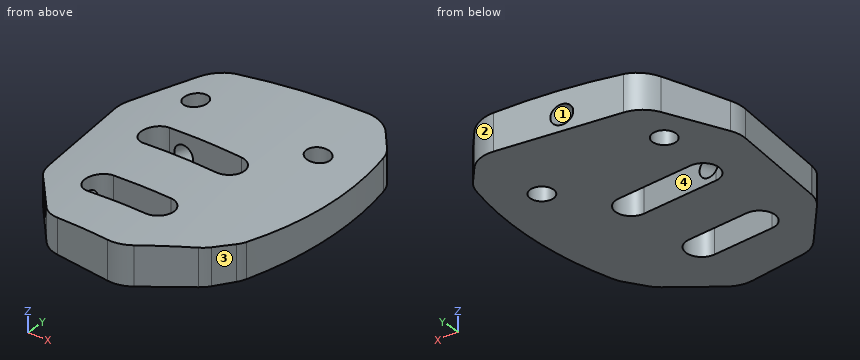
Autodesk Inventor part; units mm, degrees
ref_plane "ChannelAngleOrthoPlane" through (0.3382, 9.2918, 0) normal (-0.3338, -0.9426, 0) x (0, 0, 1)
ref_plane "YZ Plane" through (0, 0, 0) normal (1, 0, 0) x (0, 1, 0)
ref_plane "XZ Plane" through (0, 0, 0) normal (0, 1, 0) x (-1, 0, 0)
sketch "Base" plane through (0, 0, 0) normal (0, 0, 1) x (1, 0, 0)
  circle A0 centre (-15.6718, 1.2221) radius 1.5
  circle A1 centre (-13.9696, -18.0615) radius 2
  line L0 (-13.9696, -18.0615) -> (-6.0134, -18.8977) construction
  circle A2 centre (-6.0134, -18.8977) radius 2
  circle A3 centre (-14.8088, -6.9127) radius 2
  circle A4 centre (-4.8636, -7.958) radius 2
  line L1 (-14.8088, -6.9127) -> (-4.8636, -7.958) construction
  line L2 (-14.1786, -20.0505) -> (-6.2224, -20.8868)
  line L3 (-13.7605, -16.0724) -> (-5.8043, -16.9087)
  line L4 (-15.0178, -8.9017) -> (-5.0726, -9.947)
  line L5 (-14.5997, -4.9237) -> (-4.6545, -5.9689)
  line L6 (-6.0134, -18.8977) -> (-4.8636, -7.958) construction
  circle A5 centre (1.2351, -0.5549) radius 1.5
  line L7 (-15.6718, 1.2221) -> (1.2351, -0.5549) construction
  line L8 (-21.3231, -18.1609) -> (-22.5392, -2.7087)
  line L9 (-15.0979, -25.987) -> (-21.3231, -18.1609)
  line L10 (-22.5392, -2.7087) -> (-17.4079, 7.5831)
  line L11 (-17.4079, 7.5831) -> (2.5, 9.5)
  line L12 (-4.7419, -27.72) -> (2.6752, -22.6223)
  line L13 (-15.0979, -25.987) -> (-4.7419, -27.72)
  arc A6 (4.998, -19.3658) -> (6.2351, 4.8044) centre (-36.6314, -5.1184) ccw
  line L14 (2.6752, -22.6223) -> (4.998, -19.3658)
  line L15 (2.5, 9.5) -> (6.2351, 4.8044)
  line L16 (-45.5436, 0) -> (16.8418, 0) construction
  line L17 (0, -35.164) -> (0, 16.944) construction
  dimension "d119" = 8
  dimension "d129" = 10
  dimension "d290" = 11
  dimension "d293" = 3
  dimension "d294" = 122
  dimension "d295" = 123
  dimension "d296" = 149
  dimension "d297" = 146
  dimension "d298" = 138
  dimension "d299" = 136
  dimension "d300" = 160
  dimension "d301" = 44
  dimension "d302" = 94.5
  dimension "d303" = 11.5
  dimension "d304" = 20
  dimension "d305" = 15.5
  dimension "d306" = 10
  dimension "d307" = 10.5
  dimension "d308" = 9
  dimension "d309" = 4
  dimension "d310" = 6
  dimension "d311" = 6
  dimension "d312" = 8
  dimension "d313" = 17
  dimension "d314" = 2.5
  dimension "d315" = 9.5
  dimension "d316" = 11
  dimension "d317" = 8
  dimension "d318" = 5
  dimension "d319" = 4
extrude "BaseFeature" add sketch "Base" along normal blind 5
fillet "BaseFilletsFeature" radius 4 9 edges at (6.2351, 4.8044, 2.5) (2.5, 9.5, 2.5) (4.998, -19.3658, 2.5) (2.6752, -22.6223, 2.5) (-4.7419, -27.72, 2.5) (-15.0979, -25.987, 2.5) (-21.3231, -18.1609, 2.5) (-22.5392, -2.7087, 2.5) (-17.4079, 7.5831, 2.5)
sketch "SideProfile" plane through (-15.2009, 7.7956, 5) normal (-0.0958, 0.9954, 0) x (0.9954, 0.0958, 0)
  arc A0 (-8.5605, 1.5) -> (21.6674, 1) centre (8.0701, 92.9423) ccw
  line L0 (21.6674, 1) -> (21.6674, 5)
  line L1 (21.6674, 5) -> (-8.5605, 5)
  line L2 (-8.5605, 1.5) -> (-8.5605, 5)
  line L3 (15.6109, 5) -> (0, 5)
  line L4 (15.6109, 0) -> (0, 0) construction
  line L5 (-8.5605, 0) -> (-8.5605, 5)
  line L6 (21.1674, 0) -> (21.1674, 5)
  dimension "d328" = 4
  dimension "d329" = 3.5
  dimension "d330" = 0.5
extrude "SideProfileFeature" cut sketch "SideProfile" against normal through all keep common part
sketch "ChannelAngle" plane through (0, 0, 0) normal (0, 0, -1) x (-1, 0, 0)
  line L0 (18.2542, -22.019) -> (7.4314, 8.5437) construction
  line L1 (20.5618, -19.1179) -> (16.0538, -24.7853) construction
  line L2 (-0.3382, 9.2918) -> (15.2009, 7.7956) construction
  line L3 (22.4522, -3.8145) -> (21.419, -16.9417)
  dimension "d331" = 156
ref_plane "ChannelAngleOrthoPlane" through (0.3382, 9.2918, 0) normal (-0.3338, -0.9426, 0) x (0, 0, 1)
ref_plane "ChannelAngleBasePlane" through (-18.2542, -22.019, 0) normal (-0.9426, 0.3338, 0) x (0.3338, 0.9426, 0)
sketch "Channel" plane through (0.3382, 9.2918, 0) normal (-0.3338, -0.9426, 0) x (0, 0, 1)
  circle A0 centre (2, 7.4241) radius 1.25
  line L0 (0, 0) -> (0, 14.1483) construction
  line L1 (3.6483, 17.4241) -> (0, 17.4241)
  dimension "d334" = 2.5
  dimension "d335" = 2
  dimension "d336" = 10
hole "ChannelHoleFeature" at (-6.6601, 11.7701, 2) direction (-0.3338, -0.9426, 0) diameter 2.5 end through all
properties part number "ThumbRouter"
Verification items for the finished model (mm, model axes). Face numbers are marked on the shaded views. Round coordinates to 2 decimals unless told otherwise and drop trailing zeros. Use a Markdown table: item, result. Add a question column.
1. Thickness scan on probe 1 along Y at (x, z) = (-15.75, 0.3); probe 2 along Y at (x, z) = (-5, 3.2); probe 3 along Y at (x, z) = (-6.25, 0.9). Record the ranges inside material, lowest first. Write a range as [from, to].
2. Release check for a two-part mould opening along Y. For the marked faces 1, 2, 3 and 4 record: released by +Y, released by -Y, zero draft, split by the parting line, or undercut.
3. Section check A-A, the plane z = 2.1. Give the number of separate pieces and of enclosed holes in the cut face, plus the area to 3 significant figures.
4. Gauge pin test, flat ends, axial feed: pin 1 (5 mm diameter, centred on x = 1.24, y = -0.55, fed in from -Z); pin 2 (3 mm diameter, centred on x = -10, z = 3.5, fed in from -Y); pin 3 (1 mm diameter, centred on x = -15.5, z = 4.5, fed in from +Y). Record the tip position at first contact, or that the pin passes through.
Checks:
| question | item | result |
|---|---|---|
| 1 | probe 1 | y = [-25.13, -18.97], [-17.15, -8.68], [-5.15, -0.28], [2.72, 7.7] |
| 1 | probe 2 | y = [-27.45, -20.62], [-17.17, -9.95], [-5.93, 8.78] |
| 1 | probe 3 | y = [-27.47, -20.88], [-16.86, -9.82], [-5.8, 8.66] |
| 2 | face 1 | undercut |
| 2 | face 2 | released by +Y |
| 2 | face 3 | released by -Y |
| 2 | face 4 | undercut |
| 3 | separate pieces | 2 |
| 3 | enclosed holes | 2 |
| 3 | area | 726 mm^2 |
| 4 | pin 1 | stops at z = 0 |
| 4 | pin 2 | stops at y = -27.09 |
| 4 | pin 3 | stops at y = 7.81 |
